```python
from build123d import *

# Parameters (mm, degrees)
SKETCH1_W           = 45
SKETCH1_H           = 12
BOSS_EXTRUDE1_DEPTH = 8
SKETCH2_R           = 4
CUT_EXTRUDE1_DEPTH  = 8
FILLET1_R           = 4
SKETCH3_W           = 4
SKETCH3_H           = 39.830583049
CUT_EXTRUDE2_DEPTH  = 16


with BuildPart() as part:
    # Sketch1 → Boss-Extrude1 (new body)
    with BuildSketch(Plane(origin=(0, 0, 0), x_dir=(0, 0, -1), z_dir=(1, 0, 0))):
        Rectangle(SKETCH1_W, SKETCH1_H)
    extrude(amount=BOSS_EXTRUDE1_DEPTH)

    # Sketch2 → Cut-Extrude1 (cut)
    with BuildSketch(Plane(origin=(8, 0, 0), x_dir=(0, 0, -1), z_dir=(1, 0, 0))):
        with Locations((-15, 0)):
            Circle(SKETCH2_R)
        with Locations((15, 0)):
            Circle(SKETCH2_R)
    extrude(amount=-CUT_EXTRUDE1_DEPTH, mode=Mode.SUBTRACT)

    # Fillet1
    fillet1_edges = [part.edges().sort_by_distance(p)[0] for p in [
        (4, -6, -22.5),
        (4, -6, 22.5),
        (4, 6, 22.5),
        (4, 6, -22.5),
    ]]
    fillet(fillet1_edges, radius=FILLET1_R)

    # Sketch3 → Cut-Extrude2 (cut)
    with BuildSketch(Plane(origin=(0, 6, 0), x_dir=(1, 0, 0), z_dir=(0, 1, 0))):
        with Locations((2, 12.415291525)):
            Rectangle(SKETCH3_W, SKETCH3_H)
    extrude(amount=-CUT_EXTRUDE2_DEPTH, mode=Mode.SUBTRACT)


solid = part.part
```
Model file for the job. Use its own axes, mm. A direction names the side the tool comes from. Coordinates: 2 decimals unless noted, no trailing zeros. Loops run counter-clockwise (first coordinate to the right, second up) from the corner with the lowest first, then second, coordinate; pieces in that order, holes last. Notation, with made-up numbers: (5.5, 70.5) - (45.5, 70.5) arc R13 cw to (45.5, 90.5) - close; hole circle Ø5 at (73, 83). An arc over 180 degrees is marked (long way). Write item = value, one per line. Start each with the question number.
Item 1: Saw through at C-C, the plane x = 3. List the corners of the cut face in (y, z).
Item 2: Wall check: probe 1 along Y at (x, z) = (5, -15); probe 2 along Z at (x, y) = (7.5, 2.5); probe 3 along X at (y, z) = (4.25, -13.5). Give the ranges that are in metal, low to high. Write a range as [from, to].
Item 3: Saw through at A-A, the plane z = -15. List the corners of the cut face in (x, y).
Item 4: Pull direction Y, two halves, no side cores. Call faces 3 (the face through (4, 0, 19)), 4 (the face through (6.028, -4.859, -21.297)), 5 (the face through (8, 0, 0)), 6 (the face through (5, 6, 4)): +Y half, -Y half, draft (parallel to the pull), parting line (faces both ways), or undercut.
Item 5: Drop flat-ended pins along their axis: pin 1 Ø1.2 at (x, y) = (1.5, -1.5) entering from -Z; pin 2 Ø1 at (y, z) = (4, -4.5) entering from -X. Give the stop position or say it passes through.
Item 6: Saw through at D-D, the plane x = 7.5. List the corners of the cut face in (y, z).
Item 7: 3-axis set-ups, long thin cutter, end or side, ignore diameter. For faces 1 (the face through (2, 0, 7.5)), 2 (the face through (0, 3, 12)): which of +Z, -Z, +X, -X, +Y, -Y reach the whole face in a straight line?
Item 8: Saw through at B-B, the plane y = 0. List the corners of the cut face in (x, z).
Answers:
q1.outline = (-6, 7.5) - (6, 7.5) - (6, 18.5) arc R4 ccw to (2, 22.5) - (-2, 22.5) arc R4 ccw to (-6, 18.5) - close; hole circle Ø8 at (0, 15)
q2.probe_1 = [-6, -4], [4, 6]
q2.probe_2 = [-22.47, -18.12], [-11.88, 11.88], [18.12, 22.47]
q2.probe_3 = [4, 8]
q3.outline = (4, -6) - (8, -6) - (8, -4) - (4, -4) - close; (4, 4) - (8, 4) - (8, 6) - (4, 6) - close
q4.face_3 = undercut
q4.face_4 = -Y half
q4.face_5 = draft
q4.face_6 = +Y half
q5.pin_1 = 7.5
q5.pin_2 = 4
q6.outline = (-6, -18.5) arc R4 ccw to (-2, -22.5) - (2, -22.5) arc R4 ccw to (6, -18.5) - (6, 18.5) arc R4 ccw to (2, 22.5) - (-2, 22.5) arc R4 ccw to (-6, 18.5) - close; hole circle Ø8 at (0, -15); hole circle Ø8 at (0, 15)
q7.face_1 = -Z, -X, +Y, -Y
q7.face_2 = +Z, -Z, -X, +Y, -Y
q8.outline = (0, 7.5) - (4, 7.5) - (4, -11) - (8, -11) - (8, 11) - (0, 11) - close; (0, 19) - (8, 19) - (8, 22.5) - (0, 22.5) - close; (4, -22.5) - (8, -22.5) - (8, -19) - (4, -19) - close
